Geometry check sheet. Reference: the model listing, model coordinates, mm. A direction names the side the tool comes from. Give positions to 0.01 mm unless a question says otherwise; leave off trailing zeros. Loops run counter-clockwise (first coordinate to the right, second up) from the corner with the lowest first, then second, coordinate; pieces in that order, holes last. Notation, with made-up numbers: (89, 31.25) -> (110, 31.25) arc R13 cw to (110, 47.25) -> close; hole circle Ø10 at (65, 51). An arc over 180 degrees is marked (long way). Write each question's results on one line, items separated by ' | '. Start each with the question number.
1) Draft check along X on faces 4 (the face through (2.7, 2.8, -7.1)), 5 (the face through (32.218, 31.784, -23.349)), 6 (the face through (30, 34, -22)). Enter one of: pulls with the +X half, pulls with the -X half, needs draft (parallel to the pull), parting line crosses it, or undercut.
2) Depth check by flat-ended pin: pin 1 (4.5 mm diameter, centred on x = 32, y = 26, fed in from +Z); pin 2 (1.2 mm diameter, centred on x = 31.5, z = -30.5, fed in from -Y) (3 decimals); pin 3 (4 mm diameter, centred on x = 28, z = -29.5, fed in from -Y). Enter the tip coordinate at first touch or a pass-through.
3) Set-up check for faces 1 (the face through (18, 33, -13)), 2 (the face through (32.218, 31.651, -36.784)), 3 (the face through (5.297, 31.76, -58.354)): record each of +Z, -Z, +X, -X, +Y, -Y from which the full face is reachable in a straight line by a thin tool's end or side.
4) Scan lines: line 1 (Z direction, x = 4.75, y = 7); line 2 (Z direction, x = 21, y = 25); line 3 (Y direction, x = 1.5, z = -7). Record each from-to range of solid material in increasing order. Write a range as from..to.
5) Sectioned sample at C-C on x = 28. Record the cut outline in (y, z), then the cut area to 3 significant figures.
6) Sectioned sample at A-A on z = -29. Record the cut outline in (x, y) (3 decimals).
7) Sectioned sample at D-D on z = -53. Count the separate pieces of the cut face and the enclosed holes in it, then the cut area to 3 significant figures.
Autodesk Inventor part; units mm, degrees
ref_plane "YZ Plane" through (0, 0, 0) normal (1, 0, 0) x (0, 1, 0)
ref_plane "XZ Plane" through (0, 0, 0) normal (0, 1, 0) x (-1, 0, 0)
ref_plane "XY Plane" through (0, 0, 0) normal (0, 0, 1) x (1, 0, 0)
sketch "Sketch1" plane through (0, 0, 0) normal (1, 0, 0) x (0, 1, 0)
  line L0 (0, 0) -> (32.5, 0)
  line L1 (32.5, 0) -> (32.5, -13)
  line L2 (32.5, -60) -> (0, -60)
  line L3 (0, -60) -> (0, 0)
  circle A0 centre (25, -53) radius 3.3
  circle A1 centre (25, -7) radius 3.3
  circle A2 centre (7, -7) radius 3.3
  circle A3 centre (7, -53) radius 3.3
  line L4 (25, -7) -> (7, -7) construction
  line L5 (7, -7) -> (7, -53) construction
  line L6 (7, -53) -> (25, -53) construction
  line L7 (25, -53) -> (25, -7) construction
  line L8 (32.5, -13) -> (43, -13)
  line L9 (43, -13) -> (43, -47)
  line L10 (43, -47) -> (32.5, -47)
  line L11 (32.5, -47) -> (32.5, -60)
  line L12 (32.5, -13) -> (32.5, -47) construction
  circle A4 centre (25, -30) radius 6
  point P0 (32.5, -30)
  dimension "d0" = 60
  dimension "d1" = 6.6
  dimension "d2" = 18
  dimension "d3" = 46
  dimension "d4" = 25
  dimension "d5" = 32.5
  dimension "d6" = 34
  dimension "d7" = 43
  dimension "d8" = 12
extrude "Extrusion1" add sketch "Sketch1" along normal blind 25
sketch "Sketch2" plane through (25, 0, 0) normal (1, 0, 0) x (0, 0, -1)
  line L0 (47, 43) -> (13, 43)
  line L1 (13, 43) -> (13, 9)
  line L2 (13, 9) -> (47, 9)
  line L3 (47, 9) -> (47, 43)
  circle A0 centre (30, 25) radius 6
  point P0 (0, 0)
extrude "Extrusion2" add sketch "Sketch2" along normal blind 5
sketch "Sketch3" plane through (30, 0, 0) normal (1, 0, 0) x (0, 0, -1)
  circle A0 centre (30, 25) radius 6
  circle A1 centre (30, 25) radius 6
  line L0 (18.565, 27) -> (18.565, 23)
  line L1 (18.565, 23) -> (28, 13.565)
  line L2 (28, 13.565) -> (32, 13.565)
  line L3 (32, 13.565) -> (41.435, 23)
  line L4 (41.435, 23) -> (41.435, 27)
  line L5 (41.435, 27) -> (32, 36.435)
  line L6 (32, 36.435) -> (28, 36.435)
  line L7 (28, 36.435) -> (18.565, 27)
  point P0 (0, 0)
  point P1 (30, 13.565)
  point P2 (18.565, 25)
  point P3 (36.7175, 31.7175)
  point P4 (23.2825, 18.2825)
  dimension "d14" = 135
  dimension "d15" = 19
  dimension "d16" = 4
extrude "Extrusion3" add sketch "Sketch3" along normal blind 4.5
sketch "Sketch4" plane through (0, 32.5, -47) normal (0, 1, 0) x (1, 0, 0)
  circle A0 centre (6, -40) radius 5.4
  point P0 (0, -47)
  dimension "d19" = 10.8
  dimension "d20" = 6
  dimension "d21" = 7
extrude "Extrusion4" cut sketch "Sketch4" against normal blind 1.5
sketch "Sketch5" plane through (6, 31, -7) normal (0, 1, 0) x (1, 0, 0)
  circle A0 centre (0, 0) radius 3.3
  circle A1 centre (0, 0) radius 5.4 construction
  point P0 (-6, -7)
  dimension "d24" = 6.6
extrude "Extrusion5" cut sketch "Sketch5" against normal up to surface (31 mm away)
pattern_linear "Rectangular Pattern1" count 2 spacing 13 along (1, 0, 0) count 2 spacing -46 along (0, 0, 1) of "Extrusion5", "Extrusion4"
properties part number "BK10_Frame"
Result:
1) face 4: undercut | face 5: needs draft | face 6: pulls with the +X half
2) pin 1: z = -13 | pin 2: y = 13.565 | pin 3: y = 9
3) face 1: +Z, +X, +Y | face 2: -Z, +X, +Y | face 3: +Y
4) line 1: -60..-56.3, -49.7..-10.3, -3.7..0 | line 2: -60..-56.3, -49.7..-36, -24..-10.3, -3.7..0 | line 3: 0..3.7, 10.3..21.7, 28.3..31
5) outline: (9, -47) -> (43, -47) -> (43, -13) -> (9, -13) -> close; hole circle Ø12 at (25, -30) | area: 1,040 mm^2
6) outline: (0, 0) -> (25, 0) -> (25, 9) -> (30, 9) -> (30, 13.565) -> (34.5, 13.565) -> (34.5, 19.084) -> (0, 19.084) -> close; (0, 30.916) -> (34.5, 30.916) -> (34.5, 36.435) -> (30, 36.435) -> (30, 43) -> (0, 43) -> close
7) separate pieces: 9 | enclosed holes: 0 | area: 215 mm^2
